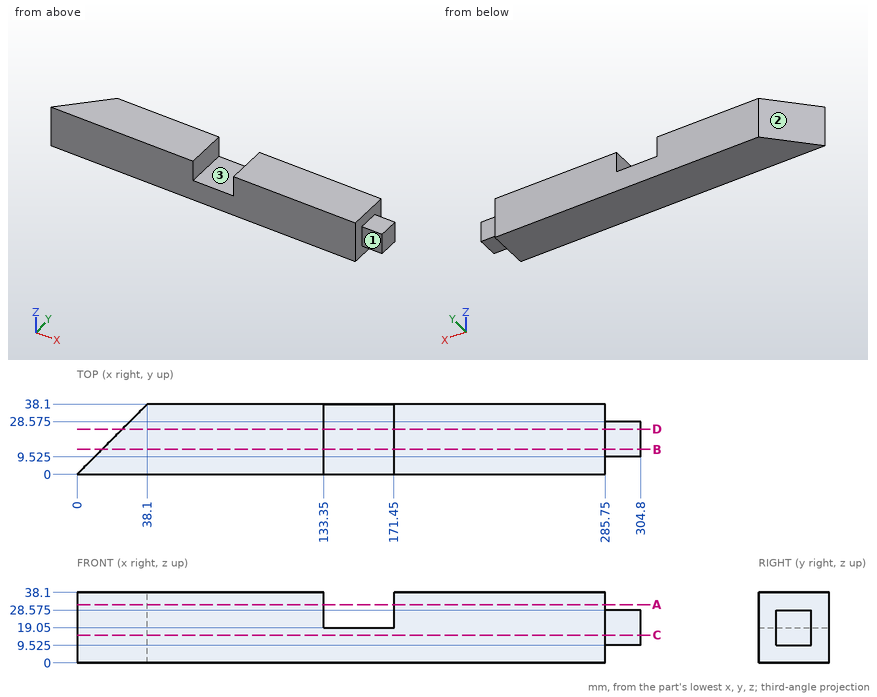
Input: dimensioned drawing with shaded views. Units: mm. Origin: part minimum x, y, z. Coordinates: 2 decimals unless noted, no trailing zeros. Write each loop counter-clockwise with the first axis right and the second up, starting at its lowest first coordinate (ties: lowest second). Pieces come first, ordered by that corner, then holes. Notation, with made-up numbers: M -39,66.5 L -18,66.5 A15 ccw -18,91.5 Z; hole C 38.25,80.5 d11. An arc over 180 degrees is marked long. Answer as a JSON object with one key per item and string values. Group by question number.
(1) Section A-A on z = 31.5. Output: boundary loops of the cut face in (x, y).
(2) Section B-B on y = 13.5. Output: boundary loops of the cut face in (x, z) (3 decimals), plus the area to 3 significant figures.
(3) Contact query for flat-ended pins moving along their axis: P1, Ø1.5, axis at y = 17.5, z = 34, coming from the +X side; P2, Ø5.5, axis at x = 291.5, z = 15, coming from the +Y side (3 decimals); P3, Ø1, axis at x = 143, y = 18.5, coming from the +Z side. Output: stop coordinate, or through.
(4) Section D-D on y = 24.5. Output: boundary loops of the cut face in (x, z) (3 decimals).
(5) Ray query, line 1 along Z through (x, y) = (165, 7); line 2 along X through (y, z) = (2, 19.5); line 3 along X through (y, z) = (8.5, 34). Return the intervals inside material, ascending. Write a range as [from, to].
(6) Mould query, pull axis X, two halves, no side actions, for the marked faces 1, 2 and 3. Classes: pulls with the +X half, pulls with the -X half, needs draft (parallel to the pull), parting line crosses it, or undercut.
(7) Section C-C on z = 15. Output: boundary loops of the cut face in (x, y) (3 decimals).
Result set:
{
 "1": {"outline": "M 0,0 L 133.35,0 L 133.35,38.1 L 38.1,38.1 Z; M 171.45,0 L 285.75,0 L 285.75,38.1 L 171.45,38.1 Z"},
 "2": {"outline": "M 13.5,0 L 285.75,0 L 285.75,9.525 L 304.8,9.525 L 304.8,28.575 L 285.75,28.575 L 285.75,38.1 L 171.45,38.1 L 171.45,19.05 L 133.35,19.05 L 133.35,38.1 L 13.5,38.1 Z", "area": "10,000 mm2"},
 "3": {"P1": "stops at x = 285.75", "P2": "stops at y = 28.575", "P3": "stops at z = 19.05"},
 "4": {"outline": "M 24.5,0 L 285.75,0 L 285.75,9.525 L 304.8,9.525 L 304.8,28.575 L 285.75,28.575 L 285.75,38.1 L 171.45,38.1 L 171.45,19.05 L 133.35,19.05 L 133.35,38.1 L 24.5,38.1 Z"},
 "5": {"line 1": "z = [0, 19.05]", "line 2": "x = [2, 133.35], [171.45, 285.75]", "line 3": "x = [8.5, 133.35], [171.45, 285.75]"},
 "6": {"face 1": "needs draft", "face 2": "pulls with the -X half", "face 3": "undercut"},
 "7": {"outline": "M 0,0 L 285.75,0 L 285.75,9.525 L 304.8,9.525 L 304.8,28.575 L 285.75,28.575 L 285.75,38.1 L 38.1,38.1 Z"}
}
